Geometry: final body of the model. Coordinates: model frame, mm. Face numbers are marked on the shaded views. Give positions to 0.01 mm unless a question says otherwise; leave off trailing zeros. Write each loop counter-clockwise with the first axis right and the second up, starting at its lowest first coordinate (ties: lowest second). Pieces come first, ordered by that corner, then holes. Notation, with made-up numbers: (44.5, 10) -> (50.5, 10) arc R23 cw to (50.5, 39) -> close; hole circle Ø4 at (75, 7.25). An arc over 180 degrees is marked (long way). Answer as a JSON object with one key per item and string values.
from build123d import *

# Parameters (mm, degrees)
F0_R     = 20
F0_R_2   = 13
F1_DEPTH = 75
F4_W     = 3
F4_H     = 9
F5_DEPTH = 75


with BuildPart() as f1:
    # F0 (on Front) → F1 (new body)
    with BuildSketch(Plane.XZ):
        Circle(F0_R)
        Circle(F0_R_2, mode=Mode.SUBTRACT)
    extrude(amount=F1_DEPTH)

    # F2 (on Right) → F3 (revolve, cut)
    with BuildSketch(Plane.YZ):
        Polygon((0, 13), (-75, 15), (-75, 13), align=None)
    revolve(axis=Axis((0, 0, 0), (0, -1, 0)), mode=Mode.SUBTRACT)

    # F4 (on face) → F5 (cut)
    with BuildSketch(Plane(origin=(0, 0, 0), x_dir=(-1, 0, 0), z_dir=(0, 1, 0))):
        with Locations((0, 16.5)):
            Rectangle(F4_W, F4_H)
    extrude(amount=-F5_DEPTH, mode=Mode.SUBTRACT)


solid = f1.part
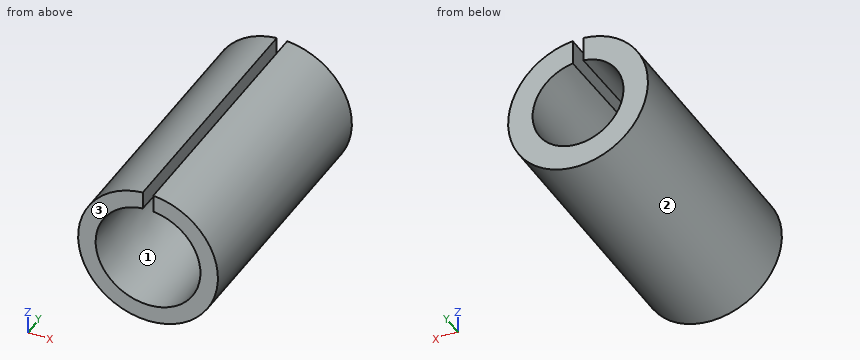
Q1. Cut plane B-B (x = 0). Return the cut outline in (y, z), and give its area (3 significant figures).
Values:
{"outline": "(-75, -20) -> (0, -20) -> (0, -13) -> (-75, -15) -> close", "area": "450 mm²"}
Q2. Cut plane C-C (y = -16). Return the cut outline in (x, z), and give its area (3 significant figures).
Values:
{"outline": "(-1.5, 13.34) -> (-1.5, 19.94) arc R20 ccw (long way) to (1.5, 19.94) -> (1.5, 13.34) arc R13.43 cw (long way) to start", "area": "671 mm²"}
Q3. First-contact query: P1, Ø10, axis at y = -47, z = 12.5, coming from the +X side; P2, Ø12, axis at y = -60.5, z = -10.5, coming from the +X side; P3, Ø8, axis at y = -47, z = -10, coming from the -X side. Flat tips, straight axial feed; report the tip coordinate or a pass-through.
Values:
{"P1": "x = 18.54", "P2": "x = 19.49", "P3": "x = -19.08"}
Q4. Mould query, pull axis X, two halves, no side actions, for the marked faces 1, 2 and 3. Classes: pulls with the +X half, pulls with the -X half, needs draft (parallel to the pull), parting line crosses it, or undercut.
Values:
{"face 1": "undercut", "face 2": "parting line crosses it", "face 3": "needs draft"}
Q5. Material intervals for L1, parallel to Z at x = 12, y = -61; L2, parallel to Z at x = 2, y = -40; L3, parallel to X at y = -46, z = 7.5, sorted ascending. Write a range as from..to.
Values:
{"L1": "-16..-8.36, 8.36..16", "L2": "-19.9..-13.92, 13.92..19.9", "L3": "-18.54..-12.09, 12.09..18.54"}
Q6. Cut plane A-A (z = 0). Return the cut outline in (x, y), and give its area (3 significant figures).
Values:
{"outline": "(-20, -75) -> (-15, -75) -> (-13, 0) -> (-20, 0) -> close; (13, 0) -> (15, -75) -> (20, -75) -> (20, 0) -> close", "area": "900 mm²"}
